Read the model definition and answer for the solid it produces. Units are mm, in the model's axes. A direction names the side the tool comes from. Give positions to 0.01 mm unless a question says otherwise; leave off trailing zeros. Order: outer loops, then holes, each group sorted by start corner. A loop starts at its lowest first (then second) coordinate and runs counter-clockwise, first axis right, second up. Notation, with made-up numbers: (48, 67) - (95, 67) arc R17 ccw to (95, 89) - close; hole circle Ø9 at (86, 0). An arc over 180 degrees is marked (long way). Use a Markdown table: item, result. Add a question column.
1. Which of the six approach directions +Z, -Z, +X, -X, +Y, -Y give full straight-line access (tool end or side, diameter ignored) to faces 1 (the cylindrical face through (30.307, 57.846, 3.287)), 2 (the cylindrical face through (30.326, 58.696, 3.287)), 3 (the flat face through (32.35, 6, 1)), 4 (the cylindrical face through (46.74, 6.46, 3.29))?
2. A cutting plane is placed at C-C on y = 6. Determine the outline of the cut face in (x, z).
3. A cutting plane is placed at B-B on y = 39. Determine the outline of the cut face in (x, z).
4. A cutting plane is placed at A-A on z = 3.2. Determine the outline of the cut face in (x, y).
5. A cutting plane is placed at D-D on x = 46.5. Determine the outline of the cut face in (y, z), and give its area (3 significant figures).
6. Flat-ended cylindrical pins translate along their axes: P1, Ø6, axis at x = 49.5, y = 25, coming from the +Z side; P2, Ø1, axis at y = 40.5, z = 3, coming from the -X side; P3, Ø1, axis at y = 28, z = 2.5, coming from the +X side. Find the tip coordinate at first contact, or state that the pin passes through.
7. Consider L1, parallel to X at y = 3.5, z = 0.4; L2, parallel to Z at x = 19, y = 35; L3, parallel to Y at x = 11, z = 2.25. Determine where each line is inside the solid, lowest interval first.
```python
from build123d import *

# Parameters (mm, degrees)
CYLINDER002_R     = 2.5
CYLINDER002_DEPTH = 5
BOX024_W          = 5
BOX024_H          = 12.5
BOX024_DEPTH      = 5
BOX001_W          = 57.7
BOX001_H          = 57.7
BOX001_DEPTH      = 0.5
BOX_W             = 59.7
BOX_H             = 59.7
BOX_DEPTH         = 1.9
BOX003_W          = 5
BOX003_H          = 22
BOX003_DEPTH      = 2.5
BOX002_W          = 5
BOX002_H          = 22
BOX002_DEPTH      = 2.5
CYLINDER001_R     = 28
CYLINDER001_DEPTH = 1.8
CYLINDER_R        = 28.85
CYLINDER_DEPTH    = 1.8


with BuildPart() as cylinder001:
    # Cylinder002 → Cylinder002 (new body)
    with BuildSketch(Plane(origin=(29.85, 12.5, 0), x_dir=(1, 0, 0), z_dir=(0, 0, 1))):
        Circle(CYLINDER002_R)
    extrude(amount=CYLINDER002_DEPTH)


with BuildPart() as cube:
    # Box024 → Box024 (new body)
    with BuildSketch(Plane(origin=(27.35, 0, 0), x_dir=(1, 0, 0), z_dir=(0, 0, 1))):
        with Locations((2.5, 6.25)):
            Rectangle(BOX024_W, BOX024_H)
    extrude(amount=BOX024_DEPTH)


with BuildPart() as layer_inside_base:
    # Box001 → Box001 (new body)
    with BuildSketch(Plane(origin=(1, 1, 1.9), x_dir=(1, 0, 0), z_dir=(0, 0, 1))):
        with Locations((28.85, 28.85)):
            Rectangle(BOX001_W, BOX001_H)
    extrude(amount=BOX001_DEPTH)


with BuildPart() as plate:
    # Box → Box (new body)
    with BuildSketch(Plane.XY):
        with Locations((29.85, 29.85)):
            Rectangle(BOX_W, BOX_H)
    extrude(amount=BOX_DEPTH)

    # Fusion: union Layer_Inside_Base
    add(layer_inside_base.part)


with BuildPart() as box003:
    # Box003 → Box003 (new body)
    with BuildSketch(Plane(origin=(54.7, 18.85, 1.9), x_dir=(1, 0, 0), z_dir=(0, 0, 1))):
        with Locations((2.5, 11)):
            Rectangle(BOX003_W, BOX003_H)
    extrude(amount=BOX003_DEPTH)


with BuildPart() as box002:
    # Box002 → Box002 (new body)
    with BuildSketch(Plane(origin=(0, 18.85, 1.9), x_dir=(1, 0, 0), z_dir=(0, 0, 1))):
        with Locations((2.5, 11)):
            Rectangle(BOX002_W, BOX002_H)
    extrude(amount=BOX002_DEPTH)


with BuildPart() as cylinder_inside:
    # Cylinder001 → Cylinder001 (new body)
    with BuildSketch(Plane(origin=(29.85, 29.85, 2.4), x_dir=(1, 0, 0), z_dir=(0, 0, 1))):
        Circle(CYLINDER001_R)
    extrude(amount=CYLINDER001_DEPTH)


with BuildPart() as cut006:
    # Cylinder → Cylinder (new body)
    with BuildSketch(Plane(origin=(29.85, 29.85, 2.4), x_dir=(1, 0, 0), z_dir=(0, 0, 1))):
        Circle(CYLINDER_R)
    extrude(amount=CYLINDER_DEPTH)

    # Cut: cut Cylinder_Inside
    add(cylinder_inside.part, mode=Mode.SUBTRACT)

    # Cut001: cut Box002
    add(box002.part, mode=Mode.SUBTRACT)

    # Cut002: cut Box003
    add(box003.part, mode=Mode.SUBTRACT)

    # Fusion001: union Plate
    add(plate.part)

    # Cut005: cut Cube
    add(cube.part, mode=Mode.SUBTRACT)

    # Cut006: cut Cylinder001
    add(cylinder001.part, mode=Mode.SUBTRACT)


solid = cut006.part
```
Output values:
| question | item | result |
|---|---|---|
| 1 | face 1 | +Z |
| 1 | face 2 | +Z, +Y |
| 1 | face 3 | +Z, -Z, -Y |
| 1 | face 4 | +Z, +X, -Y |
| 2 | outline | (0, 0) - (27.35, 0) - (27.35, 2.4) - (15.18, 2.4) - (15.18, 4.2) - (13.62, 4.2) - (13.62, 2.4) - (1, 2.4) - (1, 1.9) - (0, 1.9) - close; (32.35, 0) - (59.7, 0) - (59.7, 1.9) - (58.7, 1.9) - (58.7, 2.4) - (46.08, 2.4) - (46.08, 4.2) - (44.52, 4.2) - (44.52, 2.4) - (32.35, 2.4) - close |
| 3 | outline | (0, 0) - (59.7, 0) - (59.7, 1.9) - (58.7, 1.9) - (58.7, 2.4) - (1, 2.4) - (1, 1.9) - (0, 1.9) - close |
| 4 | outline | (3.18, 18.85) arc R28.85 ccw to (27.35, 1.11) - (27.35, 1.96) arc R28 cw to (4.1, 18.85) - close; (3.18, 40.85) - (4.1, 40.85) arc R28 cw to (55.6, 40.85) - (56.52, 40.85) arc R28.85 ccw to start; (32.35, 1.11) arc R28.85 ccw to (56.52, 18.85) - (55.6, 18.85) arc R28 cw to (32.35, 1.96) - close |
| 5 | outline | (0, 0) - (59.7, 0) - (59.7, 1.9) - (58.7, 1.9) - (58.7, 2.4) - (53.41, 2.4) - (53.41, 4.2) - (52.36, 4.2) - (52.36, 2.4) - (7.34, 2.4) - (7.34, 4.2) - (6.29, 4.2) - (6.29, 2.4) - (1, 2.4) - (1, 1.9) - (0, 1.9) - close |
| 5 | area | 146 mm² |
| 6 | P1 | z = 2.4 |
| 6 | P2 | x = 3.18 |
| 6 | P3 | x = 58.7 |
| 7 | L1 | 0 to 27.35, 32.35 to 59.7 |
| 7 | L2 | 0 to 2.4 |
| 7 | L3 | 1 to 58.7 |
